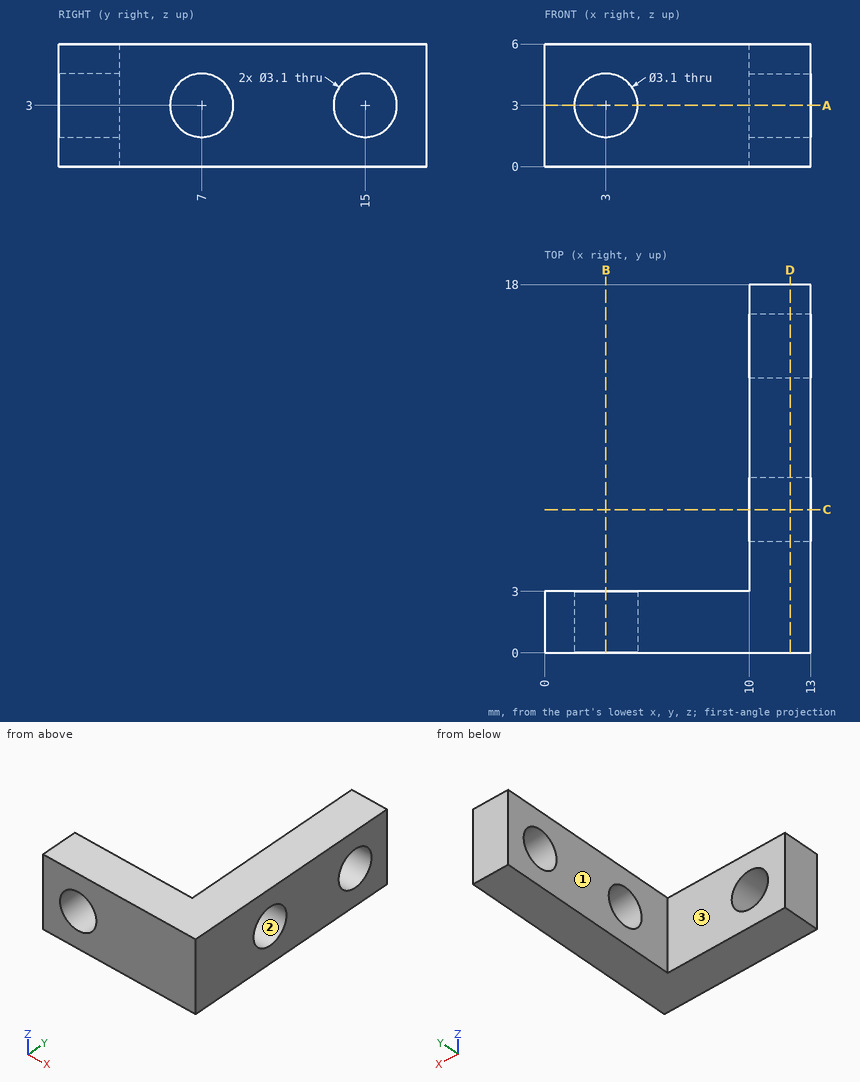
Print and shaded views of the part. All mm, measured from the part's lowest x, y and z. Round coordinates to 2 decimals unless told otherwise and drop trailing zeros. Write each loop counter-clockwise with the first axis right and the second up, starting at its lowest first coordinate (ties: lowest second). Pieces come first, ordered by that corner, then holes. Notation, with made-up numbers: (-4, 76.25) -> (47, 76.25) arc R21 ccw to (47, 114.25) -> close; hole circle Ø9 at (12, 35.5). An arc over 180 degrees is marked (long way). Answer in a Markdown table with one row per item. Add a question column.
Item 1: Mould opens along Y. For the marked faces 1, 2 and 3 say: pulls with the +Y half, pulls with the -Y half, needs draft (parallel to the pull), parting line crosses it, or undercut.
Item 2: Drill centre lines: line 1 (X direction, y = 1.5, z = 3); line 2 (Z direction, x = 12, y = 7); line 3 (Y direction, x = 11, z = 4). Where is each one in solid material? Low to high. Write a range as from..to.
Item 3: Saw through at A-A, the plane z = 3. Write the cut outline in (x, y).
Item 4: Saw through at D-D, the plane x = 12. Write the cut outline in (y, z), then the cut area to 3 significant figures.
Item 5: Saw through at C-C, the plane y = 7. Write the cut outline in (x, z).
Item 6: Saw through at B-B, the plane x = 3. Write the cut outline in (y, z).
Item 7: Drop flat-ended pins along their axis: pin 1 Ø1 at (y, z) = (11, 1.5) entering from -X; pin 2 Ø2.5 at (y, z) = (15, 3) entering from +X. Give the stop position or say it passes through.
Findings below:
| question | item | result |
|---|---|---|
| 1 | face 1 | needs draft |
| 1 | face 2 | undercut |
| 1 | face 3 | pulls with the +Y half |
| 2 | line 1 | x = 0..1.45, 4.55..13 |
| 2 | line 2 | z = 0..1.45, 4.55..6 |
| 2 | line 3 | y = 0..5.82, 8.18..13.82, 16.18..18 |
| 3 | outline | (0, 0) -> (1.45, 0) -> (1.45, 3) -> (0, 3) -> close; (4.55, 0) -> (13, 0) -> (13, 5.45) -> (10, 5.45) -> (10, 3) -> (4.55, 3) -> close; (10, 8.55) -> (13, 8.55) -> (13, 13.45) -> (10, 13.45) -> close; (10, 16.55) -> (13, 16.55) -> (13, 18) -> (10, 18) -> close |
| 4 | outline | (0, 0) -> (18, 0) -> (18, 6) -> (0, 6) -> close; hole circle Ø3.1 at (7, 3); hole circle Ø3.1 at (15, 3) |
| 4 | area | 92.9 mm^2 |
| 5 | outline | (10, 0) -> (13, 0) -> (13, 1.45) -> (10, 1.45) -> close; (10, 4.55) -> (13, 4.55) -> (13, 6) -> (10, 6) -> close |
| 6 | outline | (0, 0) -> (3, 0) -> (3, 1.45) -> (0, 1.45) -> close; (0, 4.55) -> (3, 4.55) -> (3, 6) -> (0, 6) -> close |
| 7 | pin 1 | stops at x = 10 |
| 7 | pin 2 | passes through |
